Read the model definition and answer for the solid it produces. Units are mm, in the model's axes. Give positions to 0.01 mm unless a question says otherwise; leave off trailing zeros. Write each loop counter-clockwise with the first axis right and the second up, starting at its lowest first coordinate (ties: lowest second). Pieces come first, ordered by that corner, then holes.
```python
from build123d import *

# Parameters (mm, degrees)
SKETCH1_W           = 800
SKETCH1_H           = 25
BOSS_EXTRUDE1_DEPTH = 10
SKETCH2_R           = 5.5
CUT_EXTRUDE1_DEPTH  = 20


with BuildPart() as part:
    # Sketch1 → Boss-Extrude1 (new body)
    with BuildSketch(Plane.XY):
        Rectangle(SKETCH1_W, SKETCH1_H)
    extrude(amount=BOSS_EXTRUDE1_DEPTH)

    # Sketch2 → Cut-Extrude1 (cut)
    with BuildSketch(Plane.XY):
        with Locations((370, 0)):
            Circle(SKETCH2_R)
        with Locations((-370, 0)):
            Circle(SKETCH2_R)
        Circle(SKETCH2_R)
    extrude(amount=CUT_EXTRUDE1_DEPTH, mode=Mode.SUBTRACT)


solid = part.part
```
Item 1: Section A-A (y = 0) is taken. Write down the section's boundary in (x, z), and give its area (3 significant figures).
Result set:
outline: (-400, 0) - (-375.5, 0) - (-375.5, 10) - (-400, 10) - close; (-364.5, 0) - (-5.5, 0) - (-5.5, 10) - (-364.5, 10) - close; (5.5, 0) - (364.5, 0) - (364.5, 10) - (5.5, 10) - close; (375.5, 0) - (400, 0) - (400, 10) - (375.5, 10) - close
area: 7,670 mm2
Item 2: Find the intervals of material crossed by line 1 along X through (y, z) = (0, 7); line 2 along X through (y, z) = (-1.25, 1.5); line 3 along Y through (x, z) = (0, 3.75), in increasing order.
Result set:
line 1: x = -400 to -375.5, -364.5 to -5.5, 5.5 to 364.5, 375.5 to 400
line 2: x = -400 to -375.36, -364.64 to -5.36, 5.36 to 364.64, 375.36 to 400
line 3: y = -12.5 to -5.5, 5.5 to 12.5
Item 3: This flat-tipped pin is pushed along its axis until it touches: pin 1 Ø6.5 at (x, y) = (-370, 0) entering from +Z. Where does it stop, or does it pass through?
Result set:
pin 1: passes through
